Geometry check sheet. Reference: the model listing, model coordinates, mm. Coordinates: 2 decimals unless noted, no trailing zeros. Loops run counter-clockwise (first coordinate to the right, second up) from the corner with the lowest first, then second, coordinate; pieces in that order, holes last.
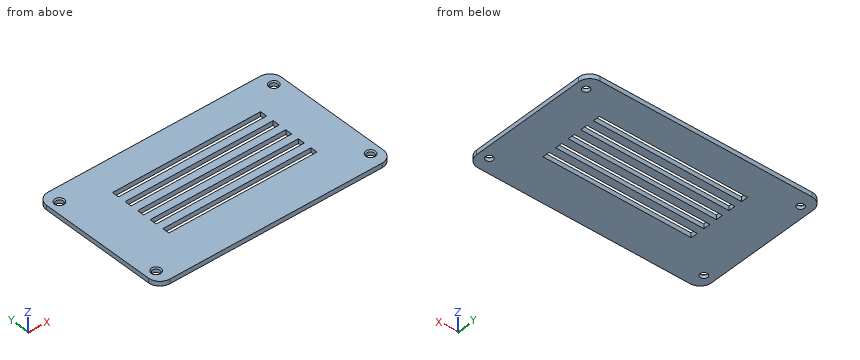
from build123d import *

# Parameters (mm, degrees)
F0_W     = 103.023604
F0_H     = 61.1
F0_R     = 1.6
F0_W_2   = 65
F0_H_2   = 3
F1_DEPTH = 2
F2_R     = 5
F3_SIZE  = 0.5


with BuildPart() as f1:
    # F0 (on Top) → F1 (new body)
    with BuildSketch(Plane.XY):
        Rectangle(F0_W, F0_H)
        with Locations((-47.05, -24.27)):
            Circle(F0_R, mode=Mode.SUBTRACT)
        with BuildLine():
            ThreePointArc((45.45, -24.27), (47.05, -22.67), (48.65, -24.27))
            ThreePointArc((48.65, -24.27), (47.05, -25.87), (45.45, -24.27))
        make_face(mode=Mode.SUBTRACT)
        with Locations((1.75037, -10.466814)):
            Rectangle(F0_W_2, F0_H_2, mode=Mode.SUBTRACT)
        with Locations((1.766913, -4.144543)):
            Rectangle(F0_W_2, F0_H_2, mode=Mode.SUBTRACT)
        with Locations((-47.05, 24.27)):
            Circle(F0_R, mode=Mode.SUBTRACT)
        with Locations((1.783457, 2.177729)):
            Rectangle(F0_W_2, F0_H_2, mode=Mode.SUBTRACT)
        with Locations((1.8, 8.5)):
            Rectangle(F0_W_2, F0_H_2, mode=Mode.SUBTRACT)
        with Locations((1.816543, 14.822271)):
            Rectangle(F0_W_2, F0_H_2, mode=Mode.SUBTRACT)
        with Locations((47.05, 24.27)):
            Circle(F0_R, mode=Mode.SUBTRACT)
    extrude(amount=F1_DEPTH)

    # F2
    f2_edges = [f1.edges().sort_by_distance(p)[0] for p in [
        (-51.511802, -30.55, 1),
        (-51.511802, 30.55, 1),
        (51.511802, -30.55, 1),
        (51.511802, 30.55, 1),
    ]]
    fillet(f2_edges, radius=F2_R)

    # F3
    f3_edges = [f1.edges().sort_by_distance(p)[0] for p in [
        (-48.65, -24.27, 2),
        (-48.65, 24.27, 2),
        (45.45, 24.27, 2),
        (48.65, -24.27, 2),
    ]]
    chamfer(f3_edges, length=F3_SIZE)


solid = f1.part
(1) Scan lines: L1, parallel to Y at x = -23, z = 1.85; L2, parallel to X at y = 8, z = 1.2; L3, parallel to Y at x = -47.05, z = 0.4. Record each from-to range of solid material in increasing order.
Findings:
L1: y = -30.55 to -11.97, -8.97 to -5.64, -2.64 to 0.68, 3.68 to 7, 10 to 13.32, 16.32 to 30.55
L2: x = -51.51 to -30.7, 34.3 to 51.51
L3: y = -30.52 to -25.87, -22.67 to 22.67, 25.87 to 30.52
(2) Sectioned sample at A-A on x = -2.5. Record the cut outline in (y, z).
Findings:
outline: (-30.55, 0) - (-11.97, 0) - (-11.97, 2) - (-30.55, 2) - close; (-8.97, 0) - (-5.64, 0) - (-5.64, 2) - (-8.97, 2) - close; (-2.64, 0) - (0.68, 0) - (0.68, 2) - (-2.64, 2) - close; (3.68, 0) - (7, 0) - (7, 2) - (3.68, 2) - close; (10, 0) - (13.32, 0) - (13.32, 2) - (10, 2) - close; (16.32, 0) - (30.55, 0) - (30.55, 2) - (16.32, 2) - close
(3) Sectioned sample at B-B on y = 24.27. Record the cut outline in (x, z).
Findings:
outline: (-51.51, 0) - (-48.65, 0) - (-48.65, 1.5) - (-49.15, 2) - (-51.51, 2) - close; (-45.45, 0) - (45.45, 0) - (45.45, 1.5) - (44.95, 2) - (-44.95, 2) - (-45.45, 1.5) - close; (48.65, 0) - (51.51, 0) - (51.51, 2) - (49.15, 2) - (48.65, 1.5) - close
(4) Sectioned sample at C-C on z = 1.15. State how many separate pieces and enclosed holes the cut face has, and give its area (3 significant figures).
Findings:
separate pieces: 1
enclosed holes: 9
area: 5,270 mm2
